Design review of the part built by this model. Coordinates are the model's own, in mm. A direction names the side the tool comes from. Coordinates: 2 decimals unless noted, no trailing zeros. Write each loop counter-clockwise with the first axis right and the second up, starting at its lowest first coordinate (ties: lowest second). Pieces come first, ordered by that corner, then holes. Notation, with made-up numbers: (74.5, 54) - (122.5, 54) arc R18 ccw to (122.5, 70) - close; hole circle Ø5 at (73.5, -1.5). An arc over 180 degrees is marked (long way). Answer as CSV lines item,"result". Start each with the question number.
Q1. For line 1 along Y through (x, z) = (23.5, 0); line 2 along Z through (x, y) = (23.5, -12); line 3 along X through (y, z) = (-25, 0.75), list the stretches that pass through material, from the lowest coordinate up. Write a range as [from, to].
Q2. Mouldability with a two-part tool opening along X and no side actions: class faces 5 (the face through (30, -6.7, -0.4)), 6 (the face through (18.568, -5.442, -0.069)), 7 (the face through (25, -23, -4.9)), 8 (the face through (20, -27, 0)) as pulls with the +X half, pulls with the -X half, needs draft (parallel to the pull), parting line crosses it, or undercut.
Q3. Machinability: for faces 1 (the face through (30, -29, 0)), 2 (the face through (20, -8.8, -4.4)), 3 (the face through (16.5, -41, 0)), 4 (the face through (22, -1, 0)), which of the approach directions +Z, -Z, +X, -X, +Y, -Y give a long, thin tool a straight path to every point of the face, cutting with its end or side? Answer none if there is none.
Q4. We need section A-A (x = 22.5). Write out the cut boundary in (y, z).
Q5. We need section B-B (x = 32). Write out the cut boundary in (y, z), plus the area to 3 significant figures.
Q6. Clearance check with flat-ended pins moving along their axes: pin 1 (3.5 mm diameter, centred on y = -40, z = -0.5, fed in from -X); pin 2 (5 mm diameter, centred on x = 27, z = -1.5, fed in from -Y); pin 3 (1.5 mm diameter, centred on y = -10, z = 4.5, fed in from -X). State where each tip first meets the part, or that it passes through.
Autodesk Inventor part; units mm, degrees
ref_plane "YZ Plane" through (0, 0, 0) normal (1, 0, 0) x (0, 1, 0)
ref_plane "XZ Plane" through (0, 0, 0) normal (0, 1, 0) x (-1, 0, 0)
ref_plane "XY Plane" through (0, 0, 0) normal (0, 0, 1) x (1, 0, 0)
sketch "Sketch1" plane through (0, 0, 0) normal (0, 0, 1) x (1, 0, 0)
  line L0 (20, -22) -> (4.1, -22) construction
  line L1 (4.1, -22) -> (4.1, -25) construction
  line L2 (4.1, -25) -> (0, -25) construction
  line L3 (30, -47) -> (20, -47) construction
  circle A0 centre (17, -17) radius 3 construction
  line L4 (14, -17) -> (14, 0) construction
  line L5 (14, 0) -> (30, 0) construction
  line L6 (20, -47) -> (20, -17) construction
  line L7 (20, -47) -> (30, -47) construction
  line L8 (30, -47) -> (30, 0) construction
  line L9 (0, -25) -> (0, 0) construction
  line L10 (30, 0) -> (30, -47) construction
  line L11 (-7.0263, 0) -> (42.1581, 0) construction
  line L12 (0, -63.6142) -> (0, 17.6853) construction
  line L13 (17, -17) -> (17, -8) construction
  circle A1 centre (17, -8) radius 3 construction
  line L14 (16.5, -38) -> (20, -38)
  line L15 (16.5, -45) -> (25, -45)
  line L16 (25, -45) -> (29.0415, -52)
  line L17 (29.0415, -52) -> (31, -52)
  line L18 (31, -52) -> (30, -44.4042)
  line L19 (30, -44.4042) -> (30, -1)
  line L20 (15, -1) -> (30, -1)
  line L21 (15, -1) -> (15, -5.7639)
  line L22 (16.5, -45) -> (16.5, -38)
  arc A2 (20, -8) -> (15, -5.7639) centre (17, -8) ccw
  line L23 (20, -8) -> (20, -38)
  line L24 (27, -1) -> (34.0711, 6.0711)
  line L25 (34.0711, 6.0711) -> (35.1317, 5.0104)
  line L26 (30, -6) -> (35.1317, 5.0104)
  point P0 (0, 0)
  point P1 (0, 0)
  dimension "d10" = 6
  dimension "d1" = 3
  dimension "d2" = 5
  dimension "d3" = 14
  dimension "d4" = 20
  dimension "d5" = 22
  dimension "d6" = 30
  dimension "d7" = 4.1
  dimension "d8" = 3
  dimension "d9" = 25
  dimension "d11" = 9
  dimension "d12" = 0
  dimension "d13" = 16
  dimension "d14" = 7
  dimension "d15" = 3.5
  dimension "d16" = 120
  dimension "d17" = 7.5
  dimension "d19" = 5
  dimension "d20" = 5
  dimension "d21" = 1
  dimension "d22" = 1
  dimension "d23" = 1
  dimension "d40" = 45
  dimension "d41" = 3
  dimension "d42" = 10
  dimension "d43" = 5
  dimension "d46" = 1.5
extrude "Extrusion1" add sketch "Sketch1" along normal mid plane 9.8
fillet "Fillet1" radius 0.5 1 edges at (15, -5.7639, 0)
fillet "Fillet2" radius 1 2 edges at (29.0415, -52, 0) (31, -52, 0)
fillet "Fillet3" radius 3 3 edges at (16.5, -45, 0) (25, -45, 0) (30, -44.4042, 0)
fillet "Fillet4" radius 2 1 edges at (15, -1, 0)
fillet "Fillet5" radius 1 1 edges at (20, -38, 0)
sketch "Sketch2" plane through (30, -44.2076, 4.9) normal (1, 0, 0) x (0, 0, -1)
  line L0 (-1.96, 44.2076) -> (11.76, 44.2076) construction
  line L1 (4.9, -19.4066) -> (4.9, 61.8929) construction
  point P0 (4.9, 44.2076)
  point P1 (4.9, 32.2076)
  dimension "d44" = 12
hole "Hole1" at (30, -12, 0) direction (-1, 0, 0) diameter 6 end through all
fillet "Fillet6" radius 2 2 edges at (30, -12, 3) (20, -12, 3)
fillet "Fillet8" radius 1 2 edges at (34.0711, 6.0711, 0) (35.1317, 5.0104, 0)
fillet "Fillet9" radius 2 1 edges at (27, -1, 0)
fillet "Fillet10" radius 1 1 edges at (16.5, -38, 0)
fillet "Fillet11" radius 2 1 edges at (30, -6, 0)
properties part number "P104" material "ABS Plastic"
Results list:
1,line 1,"y = [-45.01, -15], [-9, -1]"
1,line 2,"z = [-4.9, -3], [3, 4.9]"
1,line 3,"x = [20, 30]"
2,face 5,"pulls with the +X half"
2,face 6,"undercut"
2,face 7,"needs draft"
2,face 8,"pulls with the -X half"
3,face 1,"+Z, -Z, +X"
3,face 2,"+Z, -Z, -X"
3,face 3,"+Z, -Z, -X, -Y"
3,face 4,"+Z, -Z, -X, +Y"
4,outline,"(-45, -4.9) - (-1, -4.9) - (-1, 4.9) - (-45, 4.9) - close; hole circle Ø6 at (-12, 0)"
5,outline,"(-1.71, -4.9) - (4, -4.9) - (4, 4.9) - (-1.71, 4.9) - close"
5,area,"55.9 mm2"
6,pin 1,"stops at x = 16.5"
6,pin 2,"stops at y = -51.99"
6,pin 3,"stops at x = 20"
